Drawing for the job (mm, zero at the part's lowest x, y, z). Coordinates: 2 decimals unless noted, no trailing zeros. Loops run counter-clockwise (first coordinate to the right, second up) from the corner with the lowest first, then second, coordinate; pieces in that order, holes last.
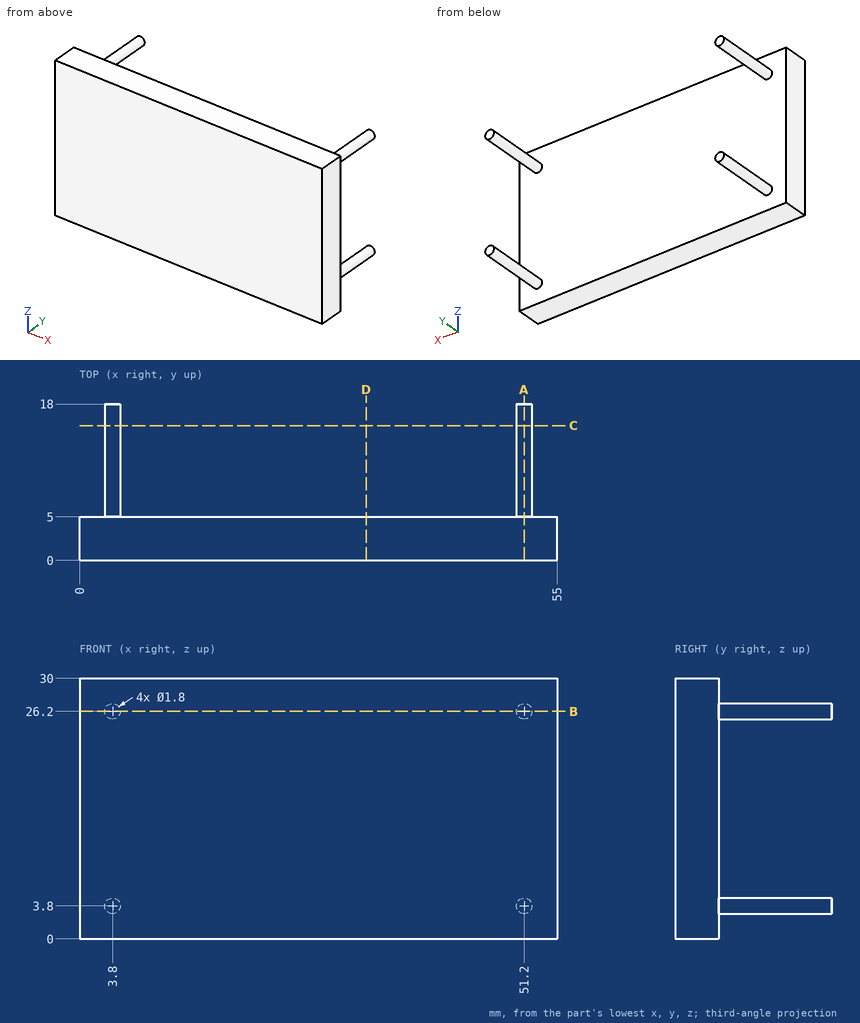
Q1. Saw through at B-B (z = 26.2). List the corners of the cut face in (x, y).
Q2. Saw through at C-C (y = 15.5). List the corners of the cut face in (x, z), plus the area to 3 significant figures.
Q3. Saw through at D-D (x = 33). List the corners of the cut face in (y, z).
Q4. Drop a flat-ended pin along its axis: P1, Ø9, axis at x = 20.5, z = 9.5, coming from the +Y side. Give the stop position or say it passes through.
Q5. Saw through at A-A (x = 51.2). List the corners of the cut face in (y, z).
Q6. Probe line 1 (Y direction, x = 10, z = 6.75); line 2 (X direction, y = 11, z = 26); line 3 (Z direction, x = 3, y = 6). List the from-to ranges inside material, lowest first.
Checked values:
1. outline: (0, 0) - (55, 0) - (55, 5) - (52.1, 5) - (52.1, 18) - (50.3, 18) - (50.3, 5) - (4.7, 5) - (4.7, 18) - (2.9, 18) - (2.9, 5) - (0, 5) - close
2. outline: circle Ø1.8 at (3.8, 3.8); circle Ø1.8 at (3.8, 26.2); circle Ø1.8 at (51.2, 3.8); circle Ø1.8 at (51.2, 26.2)
2. area: 10.2 mm2
3. outline: (0, 0) - (5, 0) - (5, 30) - (0, 30) - close
4. P1: stops at y = 5
5. outline: (0, 0) - (5, 0) - (5, 2.9) - (18, 2.9) - (18, 4.7) - (5, 4.7) - (5, 25.3) - (18, 25.3) - (18, 27.1) - (5, 27.1) - (5, 30) - (0, 30) - close
6. line 1: y = 0 to 5
6. line 2: x = 2.92 to 4.68, 50.32 to 52.08
6. line 3: z = 3.39 to 4.21, 25.79 to 26.61
